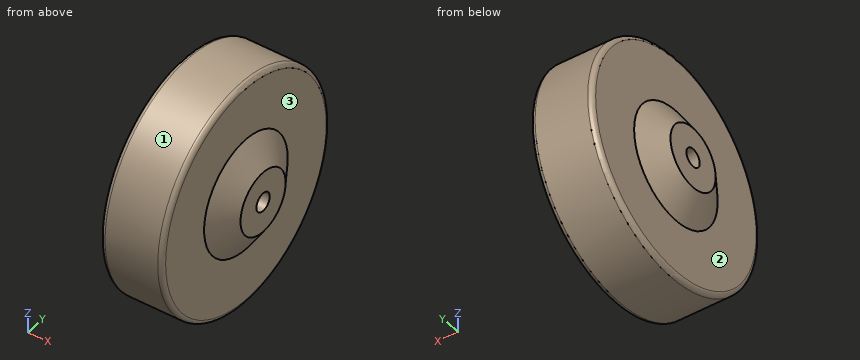
```python
from build123d import *


with BuildPart() as part:
    # Эскиз1 → Повернуть1 (revolve)
    with BuildSketch(Plane.XY):
        with BuildLine():
            Line((21, 4), (-21, 4))
            Line((-21, 4), (-21, 13.5))
            Line((-21, 13.5), (-13.5, 25))
            Line((-13.5, 25), (-13.5, 48))
            ThreePointArc((-13.5, 48), (-12.914213562, 49.414213562), (-11.5, 50))
            Line((-11.5, 50), (11.5, 50))
            ThreePointArc((11.5, 50), (12.914213562, 49.414213562), (13.5, 48))
            Line((13.5, 48), (13.5, 25))
            Line((13.5, 25), (21, 13.5))
            Line((21, 13.5), (21, 4))
        make_face()
    revolve(axis=Axis((-557.663253442, 0, 0), (1, 0, 0)))


solid = part.part
```
For this review, take the finished solid that the model builds, in its own axes (mm). Face numbers are marked on the shaded views. A direction names the side the tool comes from. Coordinates: 2 decimals unless noted, no trailing zeros. Loops run counter-clockwise (first coordinate to the right, second up) from the corner with the lowest first, then second, coordinate; pieces in that order, holes last.
1. For line 1 (Z direction, x = 0.5, y = 0); line 2 (X direction, y = 28, z = -12.5); line 3 (Z direction, x = 12, y = 0), list the stretches that pass through material, from the lowest coordinate up.
2. For the marked faces 1, 2 and 3, list the 3-axis set-ups (+Z, -Z, +X, -X, +Y, -Y) from which the entire face can be reached by the end or side of a thin tool; tool diameter is ignored.
3. Add section A-A, the plane y = 0. Give the boundary of the cut face in (x, z), then the cut area to 3 significant figures.
4. Insertion check: P1, Ø12, axis at y = 24, z = -35, coming from the -X side; P2, Ø6, axis at x = 11, y = -26.5, coming from the -Z side; P3, Ø8, axis at x = -10.5, z = -30.5, coming from the -Y side; P4, Ø5, axis at y = 0, z = 0, coming from the +X side. Each pin has a flat end and moves straight along its axis. Give the tip position at first contact, or say it passes through.
5. Add section C-C, the plane x = -7.5. Give the boundary of the cut face in (y, z).
Result:
1. line 1: z = -50 to -4, 4 to 50
1. line 2: x = -13.5 to 13.5
1. line 3: z = -49.94 to -4, 4 to 49.94
2. face 1: +X, -X
2. face 2: -X
2. face 3: +X
3. outline: (-21, -13.5) - (-13.5, -25) - (-13.5, -48) arc R2 ccw to (-11.5, -50) - (11.5, -50) arc R2 ccw to (13.5, -48) - (13.5, -25) - (21, -13.5) - (21, -4) - (-21, -4) - close; (-21, 4) - (21, 4) - (21, 13.5) - (13.5, 25) - (13.5, 48) arc R2 ccw to (11.5, 50) - (-11.5, 50) arc R2 ccw to (-13.5, 48) - (-13.5, 25) - (-21, 13.5) - close
3. area: 2,940 mm2
4. P1: stops at x = -13.5
4. P2: stops at z = -44.13
4. P3: stops at y = -42.4
4. P4: passes through
5. outline: circle Ø100 at (0, 0); hole circle Ø8 at (0, 0)
